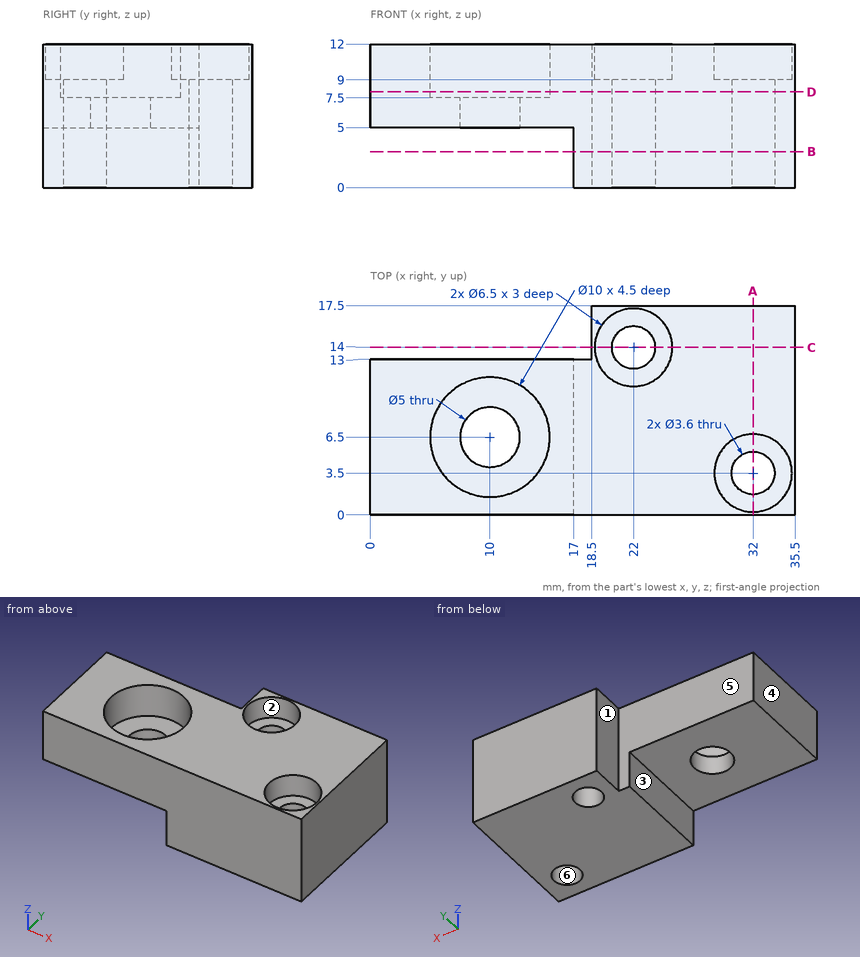
Design review of the part shown in the three views and the two pictorial views. Dimensions are in mm from the part's minimum x, y and z. A direction names the side the tool comes from. Give positions to 0.01 mm unless a question says otherwise; leave off trailing zeros. Loops run counter-clockwise (first coordinate to the right, second up) from the corner with the lowest first, then second, coordinate; pieces in that order, holes last. Notation, with made-up numbers: M 31.5,2.5 L 66.5,2.5 A14 cw 66.5,16.5 Z; hole C 9,80 d11. An arc over 180 degrees is marked long. Put each result on its own line as item: value. Start each with the question number.
(1) For pin 1 (5 mm diameter, centred on x = 11, y = 6, fed in from +Z); pin 2 (4.5 mm diameter, centred on x = 32, y = 3.5, fed in from +Z); pin 3 (3 mm diameter, centred on x = 22, y = 14, fed in from -Z); pin 4 (3.5 mm diameter, centred on x = 6.5, z = 9, fed in from +Y), all flat-tipped, find the tip position at first contact; note any pin that passes through.
(2) Add section B-B, the plane z = 3. Write out the cut boundary in (x, y), then the cut area to 3 significant figures.
(3) The part is to be moulded in two halves that separate along Y. For the marked faces 4, 5 and 6, say which applies: +Y half, -Y half, draft (parallel to the pull), parting line (faces both ways), or undercut.
(4) Add section A-A, the plane x = 32. Write out the cut boundary in (y, z), then the cut area to 3 significant figures.
(5) Add section D-D, the plane z = 8. Write out the cut boundary in (x, y), then the cut area to 3 significant figures.
(6) Machinability: for the marked faces 1, 2 and 3, which of the approach directions +Z, -Z, +X, -X, +Y, -Y give a long, thin tool a straight path to every point of the face, cutting with its end or side? Answer none if there is none.
(7) Add section C-C, the plane y = 14. Write out the cut boundary in (x, z).
(8) Wall thickness on L1, parallel to Y at x = 10, z = 5.9; L2, parallel to Y at x = 32, z = 7.25; L3, parallel to X at y = 3.75, z = 9.5: over which ranges is each line inside the solid? List them lowest first.
Result:
1. pin 1: stops at z = 7.5
1. pin 2: stops at z = 9
1. pin 3: passes through
1. pin 4: stops at y = 13
2. outline: M 17,0 L 35.5,0 L 35.5,17.5 L 18.5,17.5 L 18.5,13 L 17,13 Z; hole C 22,14 d3.6; hole C 32,3.5 d3.6
2. area: 297 mm^2
3. face 4: draft
3. face 5: +Y half
3. face 6: undercut
4. outline: M 0,0 L 1.7,0 L 1.7,9 L 0.25,9 L 0.25,12 L 0,12 Z; M 5.3,0 L 17.5,0 L 17.5,12 L 6.75,12 L 6.75,9 L 5.3,9 Z
4. area: 158 mm^2
5. outline: M 0,0 L 35.5,0 L 35.5,17.5 L 18.5,17.5 L 18.5,13 L 0,13 Z; hole C 10,6.5 d10; hole C 22,14 d3.6; hole C 32,3.5 d3.6
5. area: 439 mm^2
6. face 1: +Z, -Z, -X, +Y
6. face 2: +Z
6. face 3: -Z, -X, +Y, -Y
7. outline: M 18.5,0 L 20.2,0 L 20.2,9 L 18.75,9 L 18.75,12 L 18.5,12 Z; M 23.8,0 L 35.5,0 L 35.5,12 L 25.25,12 L 25.25,9 L 23.8,9 Z
8. L1: y = 0 to 4, 9 to 13
8. L2: y = 0 to 1.7, 5.3 to 17.5
8. L3: x = 0 to 5.82, 14.18 to 28.76, 35.24 to 35.5
